Verification items for the finished model (mm, model axes). A direction names the side the tool comes from. Round coordinates to 2 decimals unless told otherwise and drop trailing zeros. Loops run counter-clockwise (first coordinate to the right, second up) from the corner with the lowest first, then second, coordinate; pieces in that order, holes last. Notation, with made-up numbers: (9, -17.75) - (41, -17.75) arc R12 ccw to (41, 0.25) - close; hole circle Ø6 at (12.25, 8.5). An arc over 180 degrees is marked (long way). Use a Markdown table: item, result. Add a question column.
```python
from build123d import *

# Parameters (mm, degrees)
SKETCH_1_R          = 2
SKETCH_1_R_2        = 1.5
SKETCH_1_W          = 83
SKETCH_1_H          = 53
EXTRUDE_1_DEPTH     = 1.25
SKETCH_1_3_W        = 83
SKETCH_1_3_H        = 53
EXTRUDE_2_DEPTH     = 1.25
SKETCH_3_W          = 15
SKETCH_3_H          = 3
EXTRUDE_3_DEPTH     = 22
SKETCH_4_R          = 1.75
CUT_EXTRUDE_1_DEPTH = 152.167018917


with BuildPart() as part:
    # 草图1 → 凸台-拉伸1 (new, symmetric)
    with BuildSketch(Plane(origin=(0, 0, 0), x_dir=(1, 0, 0), z_dir=(0, 1, 0))):
        with BuildLine():
            Line((115, -51.818763954), (-115, -51.818763954))
            ThreePointArc((-115, -51.818763954), (-122.071067812, -48.889831766), (-125, -41.818763954))
            Line((-125, -41.818763954), (-125, 41.818763954))
            ThreePointArc((-125, 41.818763954), (-122.071067812, 48.889831766), (-115, 51.818763954))
            Line((-115, 51.818763954), (115, 51.818763954))
            ThreePointArc((115, 51.818763954), (122.071067812, 48.889831766), (125, 41.818763954))
            Line((125, 41.818763954), (125, -41.818763954))
            ThreePointArc((125, -41.818763954), (122.071067812, -48.889831766), (115, -51.818763954))
        make_face()
        with Locations(Location((120, 9.5, 0), (0, 0, 270))):
            Circle(SKETCH_1_R, mode=Mode.SUBTRACT)
        with Locations(Location((120, -9.5, 0), (0, 0, 270))):
            Circle(SKETCH_1_R, mode=Mode.SUBTRACT)
        with Locations(Location((115, 9.5, 0), (0, 0, 270))):
            Circle(SKETCH_1_R_2, mode=Mode.SUBTRACT)
        with Locations(Location((115, -9.5, 0), (0, 0, 270))):
            Circle(SKETCH_1_R_2, mode=Mode.SUBTRACT)
        with Locations(Location((-116.567558605, 9.5, 0), (0, 0, 270))):
            Circle(SKETCH_1_R_2, mode=Mode.SUBTRACT)
        with Locations(Location((-116.567558605, -9.5, 0), (0, 0, 270))):
            Circle(SKETCH_1_R_2, mode=Mode.SUBTRACT)
        with Locations(Location((-71.717926986, 42.44914331, 0), (0, 0, 270))):
            Circle(SKETCH_1_R, mode=Mode.SUBTRACT)
        with Locations(Location((3.471118404, 34.665138943, 0), (0, 0, 270))):
            Circle(SKETCH_1_R, mode=Mode.SUBTRACT)
        with Locations(Location((83.714889534, 42.44914331, 0), (0, 0, 270))):
            Circle(SKETCH_1_R, mode=Mode.SUBTRACT)
        with Locations(Location((83.714889534, -42.44914331, 0), (0, 0, 270))):
            Circle(SKETCH_1_R, mode=Mode.SUBTRACT)
        with Locations(Location((3.471118404, -34.665138943, 0), (0, 0, 270))):
            Circle(SKETCH_1_R, mode=Mode.SUBTRACT)
        with Locations(Location((-71.717926986, -42.44914331, 0), (0, 0, 270))):
            Circle(SKETCH_1_R, mode=Mode.SUBTRACT)
        with BuildLine():
            Line((-48.4, 33.818763954), (-36.4, 33.818763954))
            ThreePointArc((-36.4, 33.818763954), (-34.8, 32.218763954), (-36.4, 30.618763954))
            Line((-36.4, 30.618763954), (-48.4, 30.618763954))
            ThreePointArc((-48.4, 30.618763954), (-50, 32.218763954), (-48.4, 33.818763954))
        make_face(mode=Mode.SUBTRACT)
        with BuildLine():
            Line((-48.4, -33.818763954), (-36.4, -33.818763954))
            ThreePointArc((-36.4, -33.818763954), (-34.8, -32.218763954), (-36.4, -30.618763954))
            Line((-36.4, -30.618763954), (-48.4, -30.618763954))
            ThreePointArc((-48.4, -30.618763954), (-50, -32.218763954), (-48.4, -33.818763954))
        make_face(mode=Mode.SUBTRACT)
        with BuildLine():
            Line((48.4, -33.818763954), (36.4, -33.818763954))
            ThreePointArc((36.4, -33.818763954), (34.8, -32.218763954), (36.4, -30.618763954))
            Line((36.4, -30.618763954), (48.4, -30.618763954))
            ThreePointArc((48.4, -30.618763954), (50, -32.218763954), (48.4, -33.818763954))
        make_face(mode=Mode.SUBTRACT)
        with BuildLine():
            Line((48.4, 33.818763954), (36.4, 33.818763954))
            ThreePointArc((36.4, 33.818763954), (34.8, 32.218763954), (36.4, 30.618763954))
            Line((36.4, 30.618763954), (48.4, 30.618763954))
            ThreePointArc((48.4, 30.618763954), (50, 32.218763954), (48.4, 33.818763954))
        make_face(mode=Mode.SUBTRACT)
        with Locations((48.772829551, 0)):
            Rectangle(SKETCH_1_W, SKETCH_1_H, mode=Mode.SUBTRACT)
        with BuildLine():
            Line((-50, -41.019413621), (50, -41.019413621))
            ThreePointArc((50, -41.019413621), (51.6, -42.619413621), (50, -44.219413621))
            Line((50, -44.219413621), (-50, -44.219413621))
            ThreePointArc((-50, -44.219413621), (-51.6, -42.619413621), (-50, -41.019413621))
        make_face(mode=Mode.SUBTRACT)
        with BuildLine():
            Line((-50, 42.44914331), (50, 42.44914331))
            ThreePointArc((50, 42.44914331), (51.6, 44.04914331), (50, 45.64914331))
            Line((50, 45.64914331), (-50, 45.64914331))
            ThreePointArc((-50, 45.64914331), (-51.6, 44.04914331), (-50, 42.44914331))
        make_face(mode=Mode.SUBTRACT)
        with BuildLine():
            Line((110, 7.8731375), (110, -7.8731375))
            ThreePointArc((110, -7.8731375), (108.4, -9.4731375), (106.8, -7.8731375))
            Line((106.8, -7.8731375), (106.8, 7.8731375))
            ThreePointArc((106.8, 7.8731375), (108.4, 9.4731375), (110, 7.8731375))
        make_face(mode=Mode.SUBTRACT)
        with BuildLine():
            Line((-106.302001896, 9.756482491), (-106.302001896, -9.243517509))
            ThreePointArc((-106.302001896, -9.243517509), (-107.902001896, -10.843517509), (-109.502001896, -9.243517509))
            Line((-109.502001896, -9.243517509), (-109.502001896, 9.756482491))
            ThreePointArc((-109.502001896, 9.756482491), (-107.902001896, 11.356482491), (-106.302001896, 9.756482491))
        make_face(mode=Mode.SUBTRACT)
    extrude(amount=EXTRUDE_1_DEPTH, both=True)

    # 草图1<3> → 凸台-拉伸2 (add, symmetric)
    with BuildSketch(Plane(origin=(0, 0, 0), x_dir=(1, 0, 0), z_dir=(0, 1, 0))):
        with Locations((48.772829551, 0)):
            Rectangle(SKETCH_1_3_W, SKETCH_1_3_H)
    extrude(amount=EXTRUDE_2_DEPTH, both=True)

    # 草图3 → 凸台-拉伸3 (add)
    with BuildSketch(Plane(origin=(0, 1.25, 0), x_dir=(1, 0, 0), z_dir=(0, 1, 0))):
        with Locations((-42.391446381, -28.448620181)):
            Rectangle(SKETCH_3_W, SKETCH_3_H)
        with Locations((-42.391446381, 28.448620181)):
            Rectangle(SKETCH_3_W, SKETCH_3_H)
        with Locations((42.391446381, -28.448620181)):
            Rectangle(SKETCH_3_W, SKETCH_3_H)
        with Locations((42.391446381, 28.448620181)):
            Rectangle(SKETCH_3_W, SKETCH_3_H)
    extrude(amount=EXTRUDE_3_DEPTH)

    # 草图4 → 切除-拉伸1 (cut, through all)
    with BuildSketch(Plane.XY.offset(29.948620181)):
        with Locations((-42.391446381, 21)):
            Circle(SKETCH_4_R)
        with Locations((-42.391446381, 3.5)):
            Circle(SKETCH_4_R)
    cut_extrude_1 = extrude(amount=-CUT_EXTRUDE_1_DEPTH, mode=Mode.SUBTRACT)

    # 镜向1: 切除-拉伸1 across plane
    add(cut_extrude_1.mirror(Plane(origin=(0, 0, 0), x_dir=(0, 0, 1), z_dir=(1, 0, 0))), mode=Mode.SUBTRACT)


solid = part.part
```
Q1. Section check C-C on x = -54. Record the cut outline in (y, z), plus the area to 3 significant figures.
Q2. Thickness scan on line 1 along X through (y, z) = (0.75, -5); line 2 along Z through (x, y) = (43.5, 7); line 3 along X through (y, z) = (4.25, -28). Record the ranges inside material, lowest first.
Q3. Release check for a two-part mould opening along Z. For faces 5 (the face through (2, -1.25, -1)), 6 (the face through (-122.15, 0.02, -48.81)), 7 (the face through (42, 12, -26.949)) record: +Z half, -Z half, draft (parallel to the pull), parting line (faces both ways), or undercut.
Q4. Section check B-B on x = 21. Record the cut outline in (y, z).
Q5. Section check A-A on y = 8.5. Record the cut outline in (x, z), plus the area to 3 significant figures.
Q6. Set-up check for faces 1 (the face through (-42, 12, -29.949)), 2 (the face through (-42, 12, 29.949)), 3 (the face through (42, 12, 26.949)), 4 (the face through (122.15, 0.02, 48.81)): record each of +Z, -Z, +X, -X, +Y, -Y from which the full face is reachable in a straight line by a thin tool's end or side.
Q7. Go/stop test with flat-tipped pins: pin 1 Ø4 at (x, y) = (-42.39, 21) entering from -Z; pin 2 Ø7.5 at (x, y) = (43.5, 13.5) entering from +Z; pin 3 Ø6 at (x, z) = (-39.5, 10.5) entering from +Y. Record where each tip stops, or that it passes through.
Determined:
| question | item | result |
|---|---|---|
| 1 | outline | (-1.25, -51.82) - (1.25, -51.82) - (1.25, 51.82) - (-1.25, 51.82) - close |
| 1 | area | 259 mm² |
| 2 | line 1 | x = -125 to -109.5, -106.3 to 106.8, 110 to 125 |
| 2 | line 2 | z = -29.95 to -26.95, 26.95 to 29.95 |
| 2 | line 3 | x = -49.89 to -43.97, -40.81 to -34.89, 34.89 to 40.81, 43.97 to 49.89 |
| 3 | face 5 | draft |
| 3 | face 6 | -Z half |
| 3 | face 7 | undercut |
| 4 | outline | (-1.25, -51.82) - (1.25, -51.82) - (1.25, -45.65) - (-1.25, -45.65) - close; (-1.25, -42.45) - (1.25, -42.45) - (1.25, 41.02) - (-1.25, 41.02) - close; (-1.25, 44.22) - (1.25, 44.22) - (1.25, 51.82) - (-1.25, 51.82) - close |
| 5 | outline | (-49.89, -29.95) - (-34.89, -29.95) - (-34.89, -26.95) - (-49.89, -26.95) - close; (-49.89, 26.95) - (-34.89, 26.95) - (-34.89, 29.95) - (-49.89, 29.95) - close; (34.89, -29.95) - (49.89, -29.95) - (49.89, -26.95) - (34.89, -26.95) - close; (34.89, 26.95) - (49.89, 26.95) - (49.89, 29.95) - (34.89, 29.95) - close |
| 5 | area | 180 mm² |
| 6 | face 1 | -Z, +X, -X, +Y |
| 6 | face 2 | +Z, +X, -X, +Y |
| 6 | face 3 | +X, -X, +Y |
| 6 | face 4 | +Z, +X, +Y, -Y |
| 7 | pin 1 | stops at z = -29.95 |
| 7 | pin 2 | stops at z = 29.95 |
| 7 | pin 3 | stops at y = 1.25 |
